The drawing under review shows one solid part. Ordinate dimensions are in mm from its lowest x, y, z. Give positions to 0.01 mm unless a question says otherwise; leave off trailing zeros. Loops run counter-clockwise (first coordinate to the right, second up) from the corner with the lowest first, then second, coordinate; pieces in that order, holes last. Notation, with made-up numbers: (35.25, -37) -> (83.25, -37) arc R27 cw to (83.25, -16) -> close; hole circle Ø10 at (58, 8.25). An arc over 180 degrees is marked (long way). Answer in a Markdown table with one row per item. Add a question column.
(1) Draft analysis for pull direction Y (two halves, no side actions). For the marked faces 1, 2 and 3, state which applies: +Y half, -Y half, draft (parallel to the pull), parting line (faces both ways), or undercut.
(2) For pin 1 (3.5 mm diameter, centred on x = 25.5, y = 7.5, fed in from +Z); pin 2 (2 mm diameter, centred on x = 19.5, y = 2, fed in from +Z), all flat-tipped, find the tip position at first contact; note any pin that passes through.
(3) Consider section B-B on y = 6. Write out the cut boundary in (x, z).
(4) Consider section A-A on x = 17.5. Write out the cut boundary in (y, z), then the cut area to 3 significant figures.
(5) For line 1 (Y direction, x = 17.5, z = 3.2); line 2 (Z direction, x = 31.5, y = 5.5); line 3 (X direction, y = 5.25, z = 3.2), list the stretches that pass through material, from the lowest coordinate up.
(6) Consider section D-D on x = 26.5. Write out the cut boundary in (y, z).
(7) Consider section C-C on z = 2.95. Write out the cut boundary in (x, y).
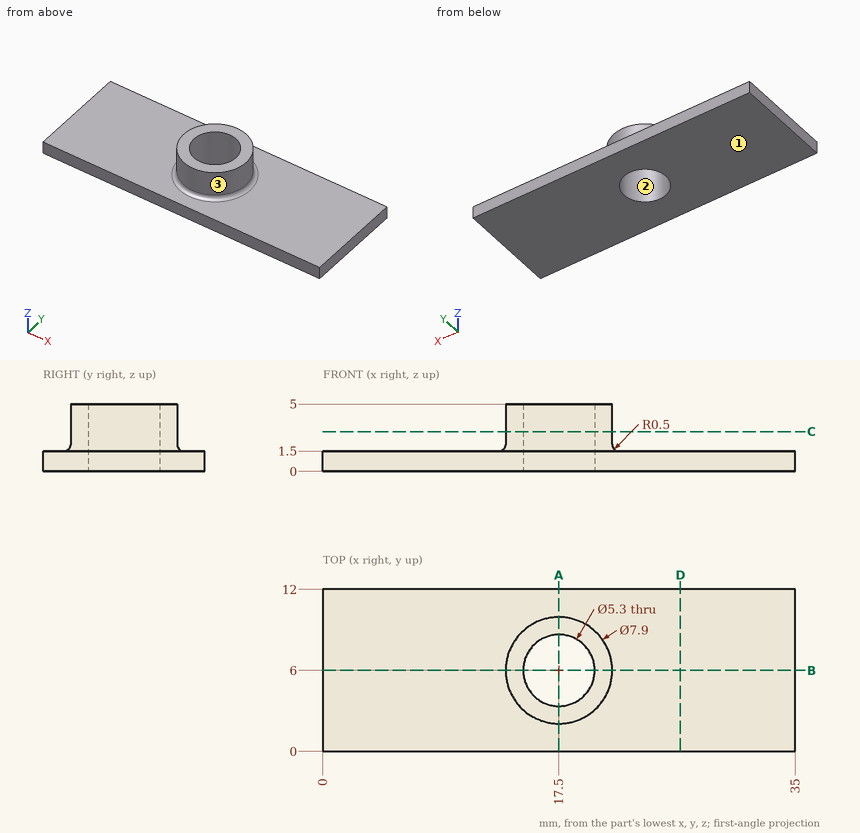
Values follow:
| question | item | result |
|---|---|---|
| 1 | face 1 | draft |
| 1 | face 2 | undercut |
| 1 | face 3 | parting line |
| 2 | pin 1 | z = 1.5 |
| 2 | pin 2 | z = 5 |
| 3 | outline | (0, 0) -> (14.85, 0) -> (14.85, 5) -> (13.55, 5) -> (13.55, 2) arc R0.5 cw to (13.05, 1.5) -> (0, 1.5) -> close; (20.15, 0) -> (35, 0) -> (35, 1.5) -> (21.95, 1.5) arc R0.5 cw to (21.45, 2) -> (21.45, 5) -> (20.15, 5) -> close |
| 4 | outline | (0, 0) -> (3.35, 0) -> (3.35, 5) -> (2.05, 5) -> (2.05, 2) arc R0.5 cw to (1.55, 1.5) -> (0, 1.5) -> close; (8.65, 0) -> (12, 0) -> (12, 1.5) -> (10.45, 1.5) arc R0.5 cw to (9.95, 2) -> (9.95, 5) -> (8.65, 5) -> close |
| 4 | area | 19.3 mm2 |
| 5 | line 1 | 2.05 to 3.35, 8.65 to 9.95 |
| 5 | line 2 | 0 to 1.5 |
| 5 | line 3 | 13.62 to 14.96, 20.04 to 21.38 |
| 6 | outline | (0, 0) -> (12, 0) -> (12, 1.5) -> (0, 1.5) -> close |
| 7 | outline | circle Ø7.9 at (17.5, 6); hole circle Ø5.3 at (17.5, 6) |
